Geometry: see drawing. Coordinates: mm, zero at the bounding-box minimum. A direction names the side the tool comes from. Give positions to 0.01 mm unless a question says otherwise; leave off trailing zeros. Order: outer loops, then holes, each group sorted by start corner. A loop starts at its lowest first (then second) coordinate and runs counter-clockwise, first axis right, second up. Notation, with made-up numbers: (87, 40) - (105, 40) arc R19 ccw to (105, 52) - close; hole circle Ø1 at (64, 23). An arc over 180 degrees is marked (long way). One line per item, written item: value.
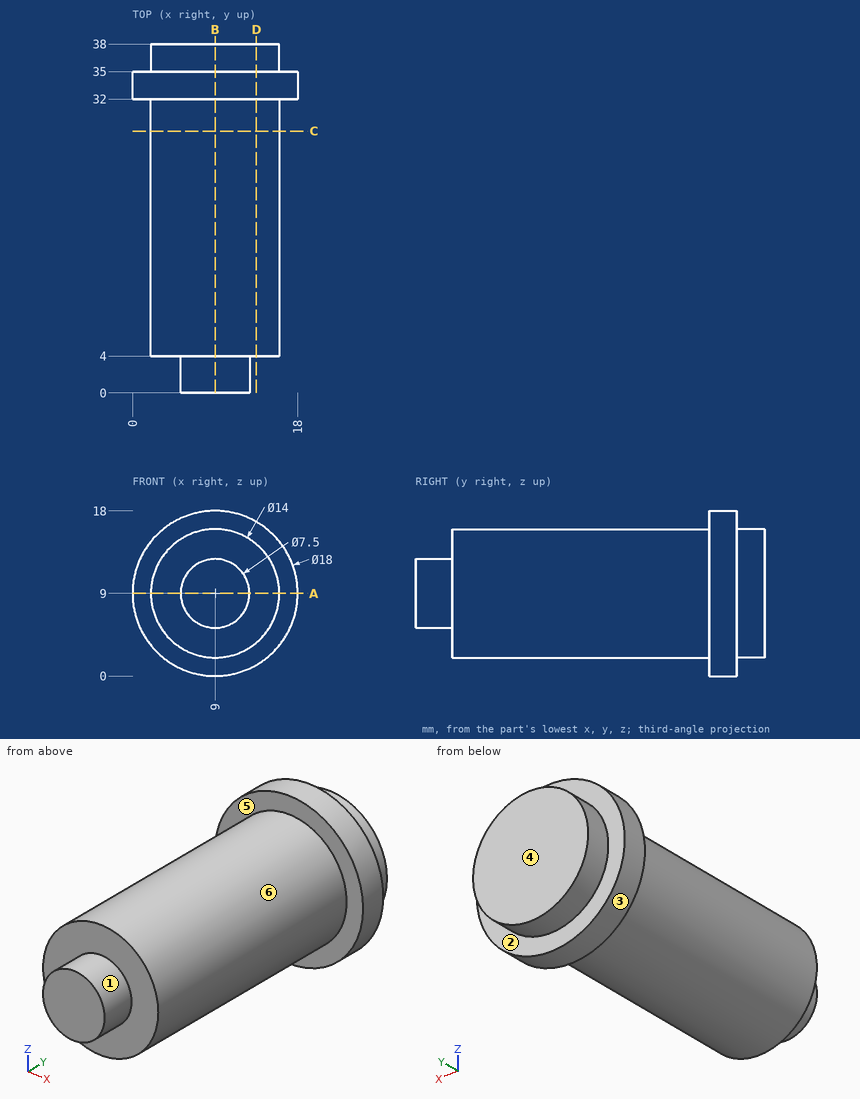
1) Mould query, pull axis Y, two halves, no side actions, for the marked faces 4, 5 and 6. Classes: released by +Y, released by -Y, zero draft, split by the parting line, or undercut.
Answers below:
face 4: released by +Y
face 5: released by -Y
face 6: zero draft
2) Set-up query: the marked faces 1, 2 and 3. Return all of +Z, -Z, +X, -X, +Y, -Y with unobstructed straight access to the full face (end or side cutting, diameter ignored); none if empty.
Answers below:
face 1: -Y
face 2: +Y
face 3: +Y, -Y
3) Section A-A, the plane z = 9. Return loops of the section in (x, y), then the cut area to 3 significant figures.
Answers below:
outline: (0, 32) - (2, 32) - (2, 4) - (5.25, 4) - (5.25, 0) - (12.75, 0) - (12.75, 4) - (16, 4) - (16, 32) - (18, 32) - (18, 35) - (16, 35) - (16, 38) - (2, 38) - (2, 35) - (0, 35) - close
area: 518 mm^2
4) Section D-D, the plane x = 13.5. Return loops of the section in (y, z).
Answers below:
outline: (4, 3.64) - (32, 3.64) - (32, 1.21) - (35, 1.21) - (35, 3.64) - (38, 3.64) - (38, 14.36) - (35, 14.36) - (35, 16.79) - (32, 16.79) - (32, 14.36) - (4, 14.36) - close
5) Section B-B, the plane x = 9. Return loops of the section in (y, z), then the cut area to 3 significant figures.
Answers below:
outline: (0, 5.25) - (4, 5.25) - (4, 2) - (32, 2) - (32, 0) - (35, 0) - (35, 2) - (38, 2) - (38, 16) - (35, 16) - (35, 18) - (32, 18) - (32, 16) - (4, 16) - (4, 12.75) - (0, 12.75) - close
area: 518 mm^2
6) First-contact query: pin 1 (6 mm diameter, centred on x = 12, y = 10, fed in from -Z); pin 2 (1 mm diameter, centred on x = 8, y = 10.5, fed in from +Z); pin 3 (5 mm diameter, centred on y = 15, z = 4.5, fed in from -X). Flat tips, straight axial feed; report the tip coordinate or a pass-through.
Answers below:
pin 1: z = 2
pin 2: z = 15.98
pin 3: x = 2.29
7) Section C-C, the plane y = 28.5. Return loops of the section in (x, z), then the cut area to 3 significant figures.
Answers below:
outline: circle Ø14 at (9, 9)
area: 154 mm^2
8) Material intervals for line 1 along Y through (x, z) = (6, 2.5); line 2 along Y through (x, z) = (15, 9.5); line 3 along X through (y, z) = (23.5, 8.75), sorted ascending.
Answers below:
line 1: 32 to 35
line 2: 4 to 38
line 3: 2 to 16
